Check sheet for the modelled part. Datum: model origin and axes. Units: mm. A direction names the side the tool comes from. Give positions to 0.01 mm unless a question says otherwise; leave off trailing zeros. Write each loop counter-clockwise with the first axis right and the second up, starting at its lowest first coordinate (ties: lowest second). Pieces come first, ordered by that corner, then holes. Notation, with made-up numbers: (65, 69.25) - (87, 69.25) arc R23 cw to (87, 85.25) - close; hole circle Ø6 at (64, 8.25). An arc over 180 degrees is marked (long way). Return JSON: item names as keys, results as strings. Group by question number.
Autodesk Inventor part; units mm, degrees
ref_plane "YZ Plane" through (0, 0, 0) normal (1, 0, 0) x (0, 1, 0)
ref_plane "XZ Plane" through (0, 0, 0) normal (0, 1, 0) x (-1, 0, 0)
ref_plane "XY Plane" through (0, 0, 0) normal (0, 0, 1) x (1, 0, 0)
sketch "Sketch1" plane through (0, 0, 0) normal (0, 0, 1) x (1, 0, 0)
  circle A0 centre (0, 0) radius 31.875
  dimension "d0" = 63.75
extrude "Extrusion1" add sketch "Sketch1" along normal blind 11
sketch "Sketch6" plane through (0, 0, 0) normal (1, 0, 0) x (0, 1, 0)
  line L0 (30.875, 8) -> (31.875, 8)
  line L1 (31.875, 8) -> (31.875, 3)
  line L2 (31.875, 3) -> (30.875, 3)
  line L3 (30.875, 3) -> (30.875, 8)
  line L4 (0, 0) -> (0, 11) construction
  line L5 (31.875, 11) -> (-31.875, 11)
  line L6 (-31.875, 0) -> (31.875, 0)
  circle A0 centre (31.875, 11) radius 1
  dimension "d62" = 1
  dimension "d63" = 5
  dimension "d65" = 31.875
  dimension "d66" = 63.75
  dimension "d67" = 3
  dimension "d81" = 2
revolve "Revolution1" cut sketch "Sketch6" angle 360 about axis through (0, 0, 0) along (0, 0, 1)
shell "Shell1" thickness 1 removed faces 1 at (5.5896, -2.5427, 0)
sketch "Sketch2" plane through (0, 0, 11) normal (0, 0, 1) x (1, 0, 0)
  circle A0 centre (0, 0) radius 31.875
  point P0 (-4, 27.5)
  point P1 (-24, -13.9)
  point P2 (24, -13.9)
  dimension "d73" = 4
  dimension "d74" = 27.5
  dimension "d77" = 13.9
  dimension "d78" = 24
  dimension "d79" = 13.9
  dimension "d80" = 24
hole "Hole1" at (-4, 27.5, 11) at (24, -13.9, 11) at (-24, -13.9, 11) direction (0, 0, -1) diameter 4 end through all
sketch "Sketch3" plane through (0, 0, 11) normal (0, 0, 1) x (1, 0, 0)
  circle A0 centre (0, 0) radius 31.875
  point P0 (-25.3, 12.7)
  dimension "d31" = 25.3
  dimension "d32" = 12.7
hole "Hole2" at (-25.3, 12.7, 11) direction (0, 0, -1) diameter 3 end through all
sketch "Sketch4" plane through (0, 0, 11) normal (0, 0, 1) x (1, 0, 0)
  point P0 (0, 0)
  point P1 (0, 3)
  dimension "d40" = 3
hole "Hole3" at (0, 3, 11) direction (0, 0, -1) diameter 12.5 end through all
sketch "Sketch5" plane through (0, 0, 11) normal (0, 0, 1) x (1, 0, 0)
  point P0 (0, 0)
  point P1 (0, -15)
  dimension "d48" = 15
hole "Hole4" at (0, -15, 11) direction (0, 0, -1) diameter 3 end through all
fillet "Fillet1" radius 1 1 edges at (0, -30.875, 11)
sketch "Sketch7" plane through (0, 0, 0) normal (0, 0, -1) x (-1, 0, 0)
  line L0 (0, 0) -> (28, 0) construction
  line L1 (28, -5) -> (28, 5) construction
  circle A0 centre (28, -5) radius 2.5
  circle A1 centre (28, 5) radius 2.5
  circle A2 centre (0, 0) radius 31.009
  dimension "d83" = 28
  dimension "d84" = 10
  dimension "d85" = 5
  dimension "d86" = 5
extrude "Extrusion2" cut sketch "Sketch7" against normal blind 2 contours A0 | A1
fillet "Fillet2" radius 2 2 edges at (-30.4611, -5.4395, 0) (-30.4611, 5.4395, 0)
equation "\"d65\" = 0.5 * d66"
properties part number "407-02" material "Stainless Steel"
Item 1: Access from +Z, -Z, +X, -X, +Y, -Y to the whole of each face (thin tool, end or side, straight path). Record for faces 4 (the face through (-26, -17, 3)), 5 (the face through (-24.725, 11.314, 10.493)), 6 (the face through (16.2, 25.3, 2)).
Item 2: Material ranges on line 1 along Y through (x, z) = (0, 10.7); line 2 along Y through (x, z) = (0, 1) (3 decimals); line 3 along Y through (x, z) = (0, 10.3), recorded low to high. Write a range as from..to.
Item 3: Mould release check, pull along Z, two halves, no side actions. Record for faces 1 (the face through (7, 0, 11)), 2 (the face through (23.399, -15.808, 10.493)), 3 (the face through (-26, -17, 8)): +Z half, -Z half, draft (parallel to the pull), parting line (faces both ways), or undercut.
Item 4: Section check A-A on z = 6. Record the cut outline in (x, y) (3 decimals), plus the area to 3 significant figures.
Item 5: Section check B-B on x = -4. Count the separate pieces of the cut face and the enclosed holes in it, plus the area to 3 significant figures.
Item 6: Depth check by flat-ended pin: pin 1 (1.5 mm diameter, centred on y = -21, z = 9, fed in from -X); pin 2 (5 mm diameter, centred on x = -4, y = 27.5, fed in from -Z); pin 3 (3 mm diameter, centred on y = 12.5, z = 7.5, fed in from +X); pin 4 (2.5 mm diameter, centred on x = 0, y = -15, fed in from +Z). Enter the tip coordinate at first touch or a pass-through.
Reply:
{
 "1": {"face 4": "none", "face 5": "+Z, -Z", "face 6": "-Z"},
 "2": {"line 1": "-30.86..-16.5, -13.5..-3.25, 9.25..30.86", "line 2": "-31.875..-30.875, 30.875..31.875", "line 3": "-31.16..-16.5, -13.5..-3.25, 9.25..31.16"},
 "3": {"face 1": "+Z half", "face 2": "draft", "face 3": "undercut"},
 "4": {"outline": "circle Ø61.75 at (0, 0); hole circle Ø59.75 at (0, 0)", "area": "191 mm²"},
 "5": {"separate pieces": "3", "enclosed holes": "0", "area": "72.7 mm²"},
 "6": {"pin 1": "x = -24.62", "pin 2": "z = 2", "pin 3": "x = 29.89", "pin 4": "through"}
}
